Design review of the part shown in the three views and the two pictorial views. Dimensions are in mm from the part's minimum x, y and z. Coordinates: 2 decimals unless noted, no trailing zeros. Loops run counter-clockwise (first coordinate to the right, second up) from the corner with the lowest first, then second, coordinate; pieces in that order, holes last. Notation, with made-up numbers: (72.5, 23) -> (113.5, 23) arc R11 ccw to (113.5, 43) -> close; hole circle Ø11 at (-27.75, -1.5). An arc over 180 degrees is marked (long way). One line per item, written item: value.
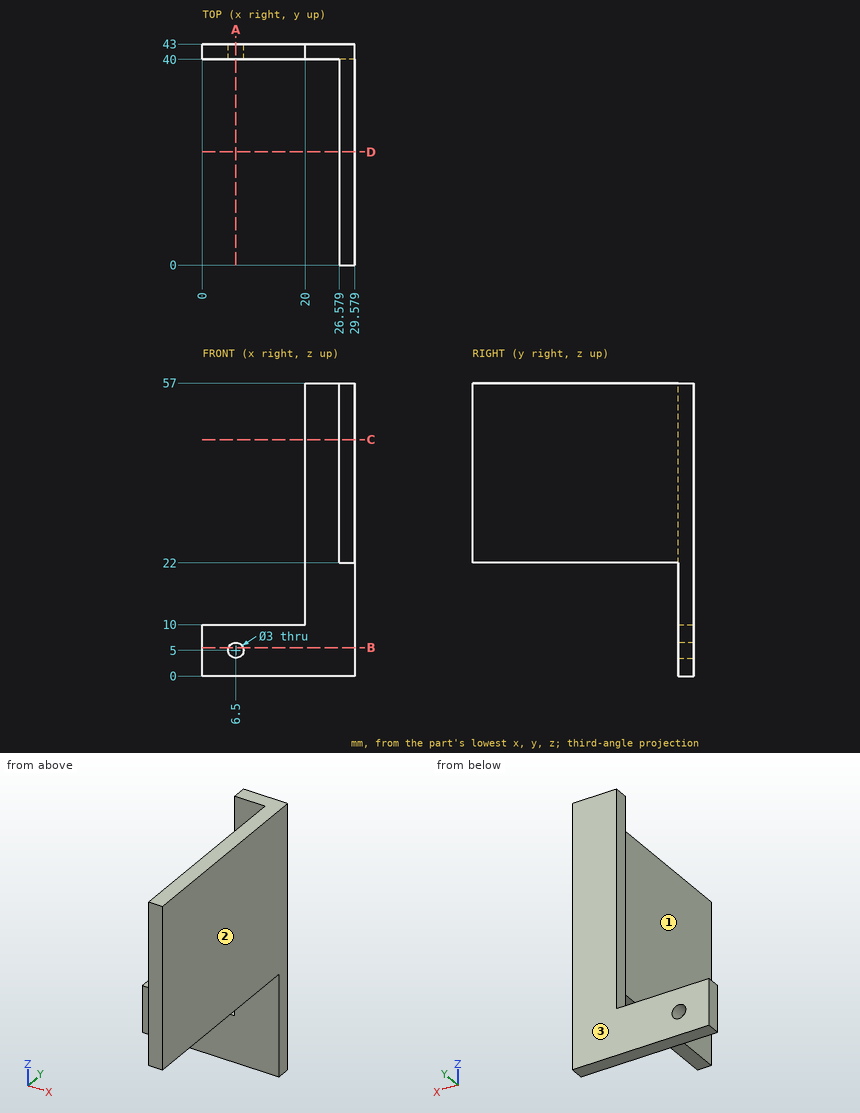
1. Take a section at A-A, the plane x = 6.5. Give the boundary of the cut face in (y, z), and give its area (3 significant figures).
Return value:
outline: (40, 0) -> (43, 0) -> (43, 3.5) -> (40, 3.5) -> close; (40, 6.5) -> (43, 6.5) -> (43, 10) -> (40, 10) -> close
area: 21.0 mm2
2. Take a section at D-D, the plane y = 22. Give the boundary of the cut face in (x, z), and give its area (3 significant figures).
Return value:
outline: (26.58, 22) -> (29.58, 22) -> (29.58, 57) -> (26.58, 57) -> close
area: 105 mm2
3. The part is to be moulded in two halves that separate along X. For the marked faces 1, 2 and 3, say which applies: pulls with the +X half, pulls with the -X half, needs draft (parallel to the pull), parting line crosses it, or undercut.
Return value:
face 1: pulls with the -X half
face 2: pulls with the +X half
face 3: needs draft
4. To check wall thickness, follow probe 1 along X at (y, z) = (41.55, 5); probe 2 along X at (y, z) = (17, 45); probe 3 along Y at (x, z) = (19.75, 9). State the ranges of each line that lie inside material, in increasing order. Write a range as from..to.
Return value:
probe 1: x = 0..5, 8..29.58
probe 2: x = 26.58..29.58
probe 3: y = 40..43
5. Take a section at B-B, the plane z = 5.5. Give the boundary of the cut face in (x, y) (1 decimal).
Return value:
outline: (0, 40) -> (5.1, 40) -> (5.1, 43) -> (0, 43) -> close; (7.9, 40) -> (29.6, 40) -> (29.6, 43) -> (7.9, 43) -> close
6. Insertion check: pin 1 Ø1 at (x, z) = (20, 14) entering from -Y; pin 2 Ø0.9 at (y, z) = (41, 42.5) entering from -X; pin 3 Ø3 at (y, z) = (31.5, 41.5) entering from -X. Each pin has a flat end and moves straight along its axis. Give the tip position at first contact, or say it passes through.
Return value:
pin 1: stops at y = 40
pin 2: stops at x = 20
pin 3: stops at x = 26.58
7. Take a section at C-C, the plane z = 46. Give the boundary of the cut face in (x, y).
Return value:
outline: (20, 40) -> (26.58, 40) -> (26.58, 0) -> (29.58, 0) -> (29.58, 43) -> (20, 43) -> close
